```python
from build123d import *

# Parameters (mm, degrees)
SKETCH1_R           = 1.98755
BOSS_EXTRUDE1_DEPTH = 1.524
SKETCH3_R           = 3.9624
SKETCH3_R_2         = 1.98755
BOSS_EXTRUDE2_DEPTH = 3.99415


with BuildPart() as part:
    # Sketch1 → Boss-Extrude1 (new body)
    with BuildSketch(Plane.XY):
        with BuildLine():
            Line((-12.7, 5.6515), (12.7, 5.6515))
            ThreePointArc((12.7, 5.6515), (18.3515, 0), (12.7, -5.6515))
            Line((12.7, -5.6515), (-12.7, -5.6515))
            ThreePointArc((-12.7, -5.6515), (-18.3515, 0), (-12.7, 5.6515))
        make_face()
        with Locations((-12.7, 0)):
            Circle(SKETCH1_R, mode=Mode.SUBTRACT)
        with Locations((12.7, 0)):
            Circle(SKETCH1_R, mode=Mode.SUBTRACT)
    boss_extrude1 = extrude(amount=BOSS_EXTRUDE1_DEPTH)

    # Sketch3 → Boss-Extrude2 (add)
    with BuildSketch(Plane(origin=(0, 0, 0), x_dir=(-1, 0, 0), z_dir=(0, 0, -1))):
        with Locations((-12.7, 0)):
            Circle(SKETCH3_R)
        with Locations((-12.7, 0)):
            Circle(SKETCH3_R_2, mode=Mode.SUBTRACT)
        with Locations((12.7, 0)):
            Circle(SKETCH3_R)
        with Locations((12.7, 0)):
            Circle(SKETCH3_R_2, mode=Mode.SUBTRACT)
    boss_extrude2 = extrude(amount=BOSS_EXTRUDE2_DEPTH)

    # Mirror4: Boss-Extrude1, Boss-Extrude2 across plane
    add(boss_extrude1.mirror(Plane.XY.offset(-3.99415)))
    add(boss_extrude2.mirror(Plane.XY.offset(-3.99415)))


solid = part.part
```
Input: part model. Units: mm. Frame: model coordinates. Give positions to 0.01 mm unless a question says otherwise; leave off trailing zeros. Loops run counter-clockwise (first coordinate to the right, second up) from the corner with the lowest first, then second, coordinate; pieces in that order, holes last. Notation, with made-up numbers: M -2,-8 L 49,-8 A19 cw 49,24 Z; hole C 57,-26 d1. An arc over 180 degrees is marked long. Answer as CSV lines item,"result". Start each with the question number.
1. Pin query (flat end, axial travel): P1, Ø3, axis at x = -12.7, y = 0, coming from the +Z side; P2, Ø5, axis at x = -7, z = -0.5, coming from the +Y side; P3, Ø4, axis at y = 4, z = -7, coming from the -X side. Return the tip coordinate at first contact, or that it passes through.
2. Pull-direction query (X, two-part tool) for faces 1 (the face through (18.35, 0.12, -8.74)), 2 (the face through (0, 0, 0)), 3 (the face through (-18.35, -0.12, -8.74)); classes: released by +X, released by -X, zero draft, split by the parting line, or undercut.
3. Section A-A on x = 6.5. Return loops of the section in (y, z).
4. Section C-C on z = -5.75. Return loops of the section in (x, y).
5. Line query: L1, parallel to Z at x = 0, y = -5; L2, parallel to Y at x = 12.7, z = -4.8; L3, parallel to X at y = 0.25, z = -6.5. Output: solid intervals per line, ascending.
6. Section B-B on y = 0. Return loops of the section in (x, z).
7. Section D-D on y = 4.5. Return loops of the section in (x, z), plus the area to 3 significant figures.
Computed values:
1,P1,"passes through"
1,P2,"stops at y = 5.65"
1,P3,"stops at x = -17.88"
2,face 1,"released by +X"
2,face 2,"undercut"
2,face 3,"released by -X"
3,outline,"M -5.65,-9.51 L 5.65,-9.51 L 5.65,-7.99 L -5.65,-7.99 Z; M -5.65,0 L 5.65,0 L 5.65,1.52 L -5.65,1.52 Z"
4,outline,"C -12.7,0 d7.92; C 12.7,0 d7.92; hole C -12.7,0 d3.98; hole C 12.7,0 d3.98"
5,L1,"z = -9.51 to -7.99, 0 to 1.52"
5,L2,"y = -3.96 to -1.99, 1.99 to 3.96"
5,L3,"x = -16.65 to -14.67, -10.73 to -8.75, 8.75 to 10.73, 14.67 to 16.65"
6,outline,"M -18.35,-9.51 L -14.69,-9.51 L -14.69,1.52 L -18.35,1.52 L -18.35,0 L -16.66,0 L -16.66,-7.99 L -18.35,-7.99 Z; M -10.71,-9.51 L 10.71,-9.51 L 10.71,1.52 L -10.71,1.52 Z; M 14.69,-9.51 L 18.35,-9.51 L 18.35,-7.99 L 16.66,-7.99 L 16.66,0 L 18.35,0 L 18.35,1.52 L 14.69,1.52 Z; hole M -8.74,-7.99 L 8.74,-7.99 L 8.74,0 L -8.74,0 Z"
7,outline,"M -16.12,-9.51 L 16.12,-9.51 L 16.12,-7.99 L -16.12,-7.99 Z; M -16.12,0 L 16.12,0 L 16.12,1.52 L -16.12,1.52 Z"
7,area,"98.3 mm²"
